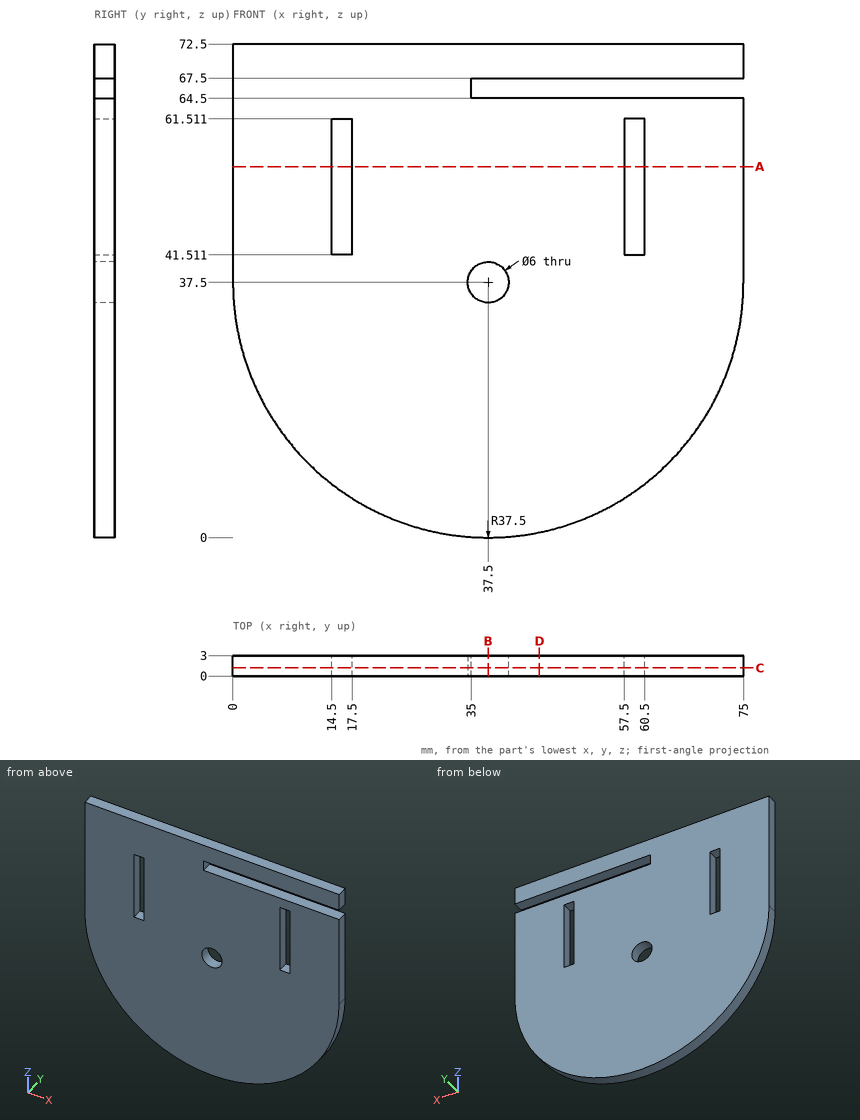
Part print with two shaded views. Sizes in mm from the minimum x, y, z corner. Round coordinates to 2 decimals unless told otherwise and drop trailing zeros. Loops run counter-clockwise (first coordinate to the right, second up) from the corner with the lowest first, then second, coordinate; pieces in that order, holes last. Notation, with made-up numbers: M 50,66 L 62,66 A12 ccw 62,83 Z; hole C 82.5,59.25 d4. An arc over 180 degrees is marked long. Put each result on its own line as item: value. Start each with the question number.
Item 1: Cut at D-D (x = 45). List the corners of the cut face in (y, z), then the cut area to 3 significant figures.
Item 2: Cut at B-B (x = 37.5). List the corners of the cut face in (y, z).
Item 3: Drill centre lines: line 1 along X through (y, z) = (1.8, 55.5); line 2 along Z through (x, y) = (37.5, 0.85); line 3 along X through (y, z) = (1.1, 37.5). Where is each one in solid material? Low to high.
Item 4: Cut at A-A (z = 54.5). List the corners of the cut face in (x, y), then the cut area to 3 significant figures.
Item 5: Drop flat-ended pins along their axis: P1, Ø1.5, axis at x = 59.5, y = 1.5, coming from the -Z side; P2, Ø0.9, axis at x = 47.5, y = 1.5, coming from the -Z side; P3, Ø1, axis at x = 40, z = 64.5, coming from the -Y side; P4, Ø0.9, axis at y = 2, z = 65.5, coming from the +X side. Give the stop position or say it passes through.
Item 6: Cut at C-C (y = 1.2). List the corners of the cut face in (x, z).
Answer block:
1. outline: M 0,0.76 L 3,0.76 L 3,64.5 L 0,64.5 Z; M 0,67.5 L 3,67.5 L 3,72.5 L 0,72.5 Z
1. area: 206 mm2
2. outline: M 0,0 L 3,0 L 3,34.5 L 0,34.5 Z; M 0,40.5 L 3,40.5 L 3,64.5 L 0,64.5 Z; M 0,67.5 L 3,67.5 L 3,72.5 L 0,72.5 Z
3. line 1: 0 to 14.5, 17.5 to 57.5, 60.5 to 75
3. line 2: 0 to 34.5, 40.5 to 64.5, 67.5 to 72.5
3. line 3: 0 to 34.5, 40.5 to 75
4. outline: M 0,0 L 14.5,0 L 14.5,3 L 0,3 Z; M 17.5,0 L 57.5,0 L 57.5,3 L 17.5,3 Z; M 60.5,0 L 75,0 L 75,3 L 60.5,3 Z
4. area: 207 mm2
5. P1: z = 6.6
5. P2: z = 1.24
5. P3: y = 0
5. P4: x = 35
6. outline: M 0,37.5 A37.5 ccw 75,37.5 L 75,64.5 L 35,64.5 L 35,67.5 L 75,67.5 L 75,72.5 L 0,72.5 Z; hole M 14.5,41.51 L 17.5,41.51 L 17.5,61.51 L 14.5,61.51 Z; hole C 37.5,37.5 d6; hole M 57.5,41.51 L 60.5,41.51 L 60.5,61.51 L 57.5,61.51 Z
